from build123d import *

# Parameters (mm, degrees)
SKETCH2_OUTSIDE_W        = 81.552
SKETCH2_OUTSIDE_H        = 81.552
SKETCH2_OUTSIDE_R        = 20
CUT_EXTRUDE_DEPTH        = 4.810952862
PATTERN_CIRCULAR_4_COUNT = 17
EXTRUDE_1_DEPTH          = 1.25


with BuildPart() as part:
    # Sketch1 → Base-Extrude (revolve)
    with BuildSketch(Plane.YZ):
        Polygon((0, -3.810952863), (-25, -3.810952863), (-31, -1.142110693), (-30.491981137, 0), (-25, -2.560952863), (0, -2.560952863), align=None)
    revolve(axis=Axis((0, 0, 5.823648763), (0, 0, -1)))

    # Sketch2 outside → Cut-Extrude (cut, through all)
    with BuildSketch(Plane(origin=(-2.40435344, 1.003568156, -3.810952862), x_dir=(-1, 0, 0), z_dir=(0, 0, -1))):
        with Locations((-2.404, -1.004)):
            Rectangle(SKETCH2_OUTSIDE_W, SKETCH2_OUTSIDE_H)
        with BuildLine():
            Line((-22.488842625, 13.883113616), (-27.712443889, 16.898961212))
            ThreePointArc((-27.712443889, 16.898961212), (-29.251140957, 14.496431844), (-30.562443889, 11.96261641))
            Line((-30.562443889, 11.96261641), (-25.338842625, 8.946768814))
            ThreePointArc((-25.338842625, 8.946768814), (19.246281655, -13.503568156), (-22.488842625, 13.883113616))
        make_face(mode=Mode.SUBTRACT)
        with Locations((-2.40435344, -1.003568156)):
            Circle(SKETCH2_OUTSIDE_R)
    extrude(amount=-CUT_EXTRUDE_DEPTH, mode=Mode.SUBTRACT)


with BuildPart() as pattern_circular_4_1:
    # Pattern Circular 4: pattern copy
    add(part.part.rotate(Axis((0, 0, 0), (0, 0, 1)), 1 * 360 / PATTERN_CIRCULAR_4_COUNT))


with BuildPart() as pattern_circular_4_2:
    # Pattern Circular 4: pattern copy
    add(part.part.rotate(Axis((0, 0, 0), (0, 0, 1)), 2 * 360 / PATTERN_CIRCULAR_4_COUNT))


with BuildPart() as pattern_circular_4_3:
    # Pattern Circular 4: pattern copy
    add(part.part.rotate(Axis((0, 0, 0), (0, 0, 1)), 3 * 360 / PATTERN_CIRCULAR_4_COUNT))


with BuildPart() as pattern_circular_4_4:
    # Pattern Circular 4: pattern copy
    add(part.part.rotate(Axis((0, 0, 0), (0, 0, 1)), 4 * 360 / PATTERN_CIRCULAR_4_COUNT))


with BuildPart() as pattern_circular_4_5:
    # Pattern Circular 4: pattern copy
    add(part.part.rotate(Axis((0, 0, 0), (0, 0, 1)), 5 * 360 / PATTERN_CIRCULAR_4_COUNT))


with BuildPart() as pattern_circular_4_6:
    # Pattern Circular 4: pattern copy
    add(part.part.rotate(Axis((0, 0, 0), (0, 0, 1)), 6 * 360 / PATTERN_CIRCULAR_4_COUNT))


with BuildPart() as pattern_circular_4_7:
    # Pattern Circular 4: pattern copy
    add(part.part.rotate(Axis((0, 0, 0), (0, 0, 1)), 7 * 360 / PATTERN_CIRCULAR_4_COUNT))


with BuildPart() as pattern_circular_4_8:
    # Pattern Circular 4: pattern copy
    add(part.part.rotate(Axis((0, 0, 0), (0, 0, 1)), 8 * 360 / PATTERN_CIRCULAR_4_COUNT))


with BuildPart() as pattern_circular_4_9:
    # Pattern Circular 4: pattern copy
    add(part.part.rotate(Axis((0, 0, 0), (0, 0, 1)), 9 * 360 / PATTERN_CIRCULAR_4_COUNT))


with BuildPart() as pattern_circular_4_10:
    # Pattern Circular 4: pattern copy
    add(part.part.rotate(Axis((0, 0, 0), (0, 0, 1)), 10 * 360 / PATTERN_CIRCULAR_4_COUNT))


with BuildPart() as pattern_circular_4_11:
    # Pattern Circular 4: pattern copy
    add(part.part.rotate(Axis((0, 0, 0), (0, 0, 1)), 11 * 360 / PATTERN_CIRCULAR_4_COUNT))


with BuildPart() as pattern_circular_4_12:
    # Pattern Circular 4: pattern copy
    add(part.part.rotate(Axis((0, 0, 0), (0, 0, 1)), 12 * 360 / PATTERN_CIRCULAR_4_COUNT))


with BuildPart() as pattern_circular_4_13:
    # Pattern Circular 4: pattern copy
    add(part.part.rotate(Axis((0, 0, 0), (0, 0, 1)), 13 * 360 / PATTERN_CIRCULAR_4_COUNT))


with BuildPart() as pattern_circular_4_14:
    # Pattern Circular 4: pattern copy
    add(part.part.rotate(Axis((0, 0, 0), (0, 0, 1)), 14 * 360 / PATTERN_CIRCULAR_4_COUNT))


with BuildPart() as pattern_circular_4_15:
    # Pattern Circular 4: pattern copy
    add(part.part.rotate(Axis((0, 0, 0), (0, 0, 1)), 15 * 360 / PATTERN_CIRCULAR_4_COUNT))


with BuildPart() as pattern_circular_4_16:
    # Pattern Circular 4: pattern copy
    add(part.part.rotate(Axis((0, 0, 0), (0, 0, 1)), 16 * 360 / PATTERN_CIRCULAR_4_COUNT))


with BuildPart() as part_1:
    add(part.part)

    add(pattern_circular_4_1.part)  # Extrude 1 merges Pattern Circular 4_1

    add(pattern_circular_4_2.part)  # Extrude 1 merges Pattern Circular 4_2

    add(pattern_circular_4_3.part)  # Extrude 1 merges Pattern Circular 4_3

    add(pattern_circular_4_4.part)  # Extrude 1 merges Pattern Circular 4_4

    add(pattern_circular_4_5.part)  # Extrude 1 merges Pattern Circular 4_5

    add(pattern_circular_4_6.part)  # Extrude 1 merges Pattern Circular 4_6

    add(pattern_circular_4_7.part)  # Extrude 1 merges Pattern Circular 4_7

    add(pattern_circular_4_8.part)  # Extrude 1 merges Pattern Circular 4_8

    add(pattern_circular_4_9.part)  # Extrude 1 merges Pattern Circular 4_9

    add(pattern_circular_4_10.part)  # Extrude 1 merges Pattern Circular 4_10

    add(pattern_circular_4_11.part)  # Extrude 1 merges Pattern Circular 4_11

    add(pattern_circular_4_12.part)  # Extrude 1 merges Pattern Circular 4_12

    add(pattern_circular_4_13.part)  # Extrude 1 merges Pattern Circular 4_13

    add(pattern_circular_4_14.part)  # Extrude 1 merges Pattern Circular 4_14

    add(pattern_circular_4_15.part)  # Extrude 1 merges Pattern Circular 4_15

    add(pattern_circular_4_16.part)  # Extrude 1 merges Pattern Circular 4_16
    # Sketch 2 → Extrude 1 (add)
    with BuildSketch(Plane.XY.offset(-2.560952863)):
        with BuildLine():
            Line((1.916994129, 17.651490971), (1.777021869, 19.920898405))
            ThreePointArc((1.777021869, 19.920898405), (-1.231218123, 19.962066575), (-4.211598103, 19.551532969))
            Line((-4.211598103, 19.551532969), (-4.071625844, 17.282125534))
            Line((-4.071625844, 17.282125534), (1.916994129, 17.651490971))
        make_face()
    extrude(amount=-EXTRUDE_1_DEPTH)


solid = part_1.part
The listing builds one solid part. Answer for the finished solid, in the listing's coordinates (mm). A direction names the side the tool comes from. Coordinates: 2 decimals unless noted, no trailing zeros. Write each loop counter-clockwise with the first axis right and the second up, starting at its lowest first coordinate (ties: lowest second). Pieces come first, ordered by that corner, then holes. Notation, with made-up numbers: (53, 23) - (112, 23) arc R17 ccw to (112, 54) - close; hole circle Ø8 at (-36, 38). An arc over 180 degrees is marked (long way). Put each result on its own line as item: value.
1. Flat-ended cylindrical pins translate along their axes: pin 1 Ø2 at (x, z) = (-18.5, -2.5) entering from +Y; pin 2 Ø15 at (x, y) = (6.5, -7.5) entering from +Z. Find the tip coordinate at first contact, or state that the pin passes through.
Answer sheet:
pin 1: stops at y = 22.56
pin 2: passes through
2. Find the intervals of material crossed by line 1 along Z through (x, y) = (18.5, -11); line 2 along Y through (x, z) = (0, -2.9); line 3 along Y through (x, z) = (0, -3.3), in increasing order. Write a range as from..to.
Answer sheet:
line 1: z = -3.81..-2.56
line 2: y = -25..-20, 17.53..27.05
line 3: y = -25..-20, 17.53..26.15
3. Determine the mould class of faces 1 (the face through (-3.36, -27.5, -1.3)), 2 (the face through (17.545, 21.875, -2.458)), 3 (the face through (27.37, 4.29, -1.3)), 4 (the face through (-21.266, -18.279, -2.458)) for opening direction X: pulls with the +X half, pulls with the -X half, needs draft (parallel to the pull), parting line crosses it, or undercut.
Answer sheet:
face 1: undercut
face 2: pulls with the +X half
face 3: undercut
face 4: pulls with the -X half
4. The part is cut by section A-A on y = 0. Give the vertices of the cut face in (x, z).
Answer sheet:
outline: (-31, -1.14) - (-25, -3.81) - (-20, -3.81) - (-20, -2.56) - (-25, -2.56) - (-30.49, 0) - close; (20, -3.81) - (25, -3.81) - (25, -2.56) - (20, -2.56) - close
5. The part is cut by section B-B on z = -1.9. State how many separate pieces and enclosed holes the cut face has, plus the area to 3 significant figures.
Answer sheet:
separate pieces: 17
enclosed holes: 0
area: 279 mm^2
6. A tool of negligible diameter and unlimited length cuts with its end or side. For faces 5 (the face through (16.04, -22.59, -1.3)), 6 (the face through (-15.654, -19.492, -3.195)), 7 (the face through (27.974, 1.458, -1.914)), 8 (the face through (-0.565, -27.756, -1.914)), from which of +Z, -Z, +X, -X, +Y, -Y can it reach the whole face along a straight path? Write none if from no direction.
Answer sheet:
face 5: +Z
face 6: +Z, -Z
face 7: +Z, -Z, +X
face 8: +Z, -Z, -Y
